Verification items for the finished model (mm, model axes). A direction names the side the tool comes from. Round coordinates to 2 decimals unless told otherwise and drop trailing zeros. Write each loop counter-clockwise with the first axis right and the second up, starting at its lowest first coordinate (ties: lowest second). Pieces come first, ordered by that corner, then holes. Notation, with made-up numbers: (-12.75, -24.5) - (16.25, -24.5) arc R29 cw to (16.25, -4.5) - close; hole circle Ø6 at (61, -39). An arc over 180 degrees is marked (long way). Answer as a JSON object with one key per item and string values.
```python
from build123d import *

# Parameters (mm, degrees)
F0_W     = 100.019608
F0_H     = 91
F2_DEPTH = 3
F3_DEPTH = 10
F4_R     = 8


with BuildPart() as f2:
    # F0 (on Front) → F2 (new body)
    with BuildSketch(Plane.XZ):
        with Locations((0, 25.5)):
            Rectangle(F0_W, F0_H)
        Polygon((0, 0), (-29.386316, 0), (-31.587102, -4.489604), (-32.485023, -4.049446), (-30.5, 0), (-31.613684, 0), (-35.009804, 0), (-35.009804, 1), (-30.009804, 1), (-5.990196, 50), (-10.5, 50), (-10.5, 51), (-5.5, 51), (-5.009804, 52), (-3.299214, 55.489604), (-2.401293, 55.049446), (-4.386316, 51), (0, 51), (4.386316, 51), (2.401293, 55.049446), (3.299214, 55.489604), (5.009804, 52), (5.5, 51), (10.5, 51), (10.5, 50), (5.990196, 50), (30.009804, 1), (35.009804, 1), (35.009804, 0), (31.613684, 0), (30.5, 0), (32.485023, -4.049446), (31.587102, -4.489604), (29.386316, 0), align=None, mode=Mode.SUBTRACT)
    extrude(amount=-F2_DEPTH)

    # F1 (on face) → F3 (join)
    with BuildSketch(Plane.XZ):
        with BuildLine():
            Line((-35.334654, -17), (-33.334654, -17))
            ThreePointArc((-33.334654, -17), (-35.804867, -5.945831), (-47.009804, -4.288724))
            Line((-47.009804, -4.288724), (-47.009804, -6.288724))
            ThreePointArc((-47.009804, -6.288724), (-37.230822, -7.34828), (-35.334654, -17))
        make_face()
        with BuildLine():
            ThreePointArc((-47.009804, 55.288724), (-35.804867, 56.945831), (-33.334654, 68))
            Line((-33.334654, 68), (-35.334654, 68))
            ThreePointArc((-35.334654, 68), (-37.230822, 58.34828), (-47.009804, 57.288724))
            Line((-47.009804, 57.288724), (-47.009804, 55.288724))
        make_face()
        with BuildLine():
            Line((35.334654, 68), (33.334654, 68))
            ThreePointArc((33.334654, 68), (35.804867, 56.945831), (47.009804, 55.288724))
            Line((47.009804, 55.288724), (47.009804, 57.288724))
            ThreePointArc((47.009804, 57.288724), (37.230822, 58.34828), (35.334654, 68))
        make_face()
        with BuildLine():
            ThreePointArc((47.009804, -4.288724), (35.804867, -5.945831), (33.334654, -17))
            Line((33.334654, -17), (35.334654, -17))
            ThreePointArc((35.334654, -17), (37.230822, -7.34828), (47.009804, -6.288724))
            Line((47.009804, -6.288724), (47.009804, -4.288724))
        make_face()
    extrude(amount=F3_DEPTH)

    # F4
    f4_edges = [f2.edges().sort_by_distance(p)[0] for p in [
        (-50.009804, 1.5, 71),
        (50.009804, 1.5, 71),
        (50.009804, 1.5, -20),
        (-50.009804, 1.5, -20),
    ]]
    fillet(f4_edges, radius=F4_R)


solid = f2.part
```
1. Cross-section at C-C (z = 47). Record the boundary of the cut face in (x, y).
Completed:
{"outline": "(-50.01, 0) - (-7.46, 0) - (-7.46, 3) - (-50.01, 3) - close; (7.46, 0) - (50.01, 0) - (50.01, 3) - (7.46, 3) - close"}
2. Access from +Z, -Z, +X, -X, +Y, -Y to the whole of each face (thin tool, end or side, straight path). Record for faces 1 (the face through (36.6, -10, -7.6)), 2 (the face through (35.93, -4.93, -5.83)), 3 (the face through (-31.506, 1.479, -2.053)).
Completed:
{"face 1": "+Z, -Z, +X, -X, -Y", "face 2": "-Y", "face 3": "+Y, -Y"}
3. Mould release check, pull along X, two halves, no side actions. Record for faces 4 (the face through (-47.73, 1.52, -17.59)), 5 (the face through (33, 1, 0)), 6 (the face through (-37, -10, -7)): released by +X, released by -X, zero draft, split by the parting line, or undercut.
Completed:
{"face 4": "released by -X", "face 5": "undercut", "face 6": "zero draft"}
4. Cross-section at A-A (y = -6.5). Record the boundary of the cut face in (x, z).
Completed:
{"outline": "(-47.01, -6.29) arc R8.3 cw to (-35.33, -17) - (-33.33, -17) arc R10 ccw to (-47.01, -4.29) - close; (-47.01, 55.29) arc R10 ccw to (-33.33, 68) - (-35.33, 68) arc R8.3 cw to (-47.01, 57.29) - close; (33.33, -17) - (35.33, -17) arc R8.3 cw to (47.01, -6.29) - (47.01, -4.29) arc R10 ccw to start; (33.33, 68) arc R10 ccw to (47.01, 55.29) - (47.01, 57.29) arc R8.3 cw to (35.33, 68) - close"}
5. Material ranges on probe 1 along Y at (x, z) = (29.5, 50); probe 2 along Z at (x, y) = (5, 0.75); probe 3 along X at (y, z) = (-1.75, -15), recorded low to high. Write a range as from..to.
Completed:
{"probe 1": "y = 0..3", "probe 2": "z = -20..0, 52.02..71", "probe 3": "x = -34.69..-32.76, 32.76..34.69"}
6. Go/stop test with flat-tipped pins: pin 1 (0.6 mm diameter, centred on y = -3.5, z = 56.5, fed in from -X); pin 2 (2 mm diameter, centred on y = -7.5, z = 56, fed in from +X); pin 3 (1.6 mm diameter, centred on x = -34, y = -6.5, fed in from -Z); pin 4 (3 mm diameter, centred on y = -0.5, z = -6.5, fed in from +X). Record where each tip stops, or that it passes through.
Completed:
{"pin 1": "stops at x = -47.01", "pin 2": "stops at x = 47.01", "pin 3": "stops at z = -17", "pin 4": "stops at x = 50.01"}
7. Cross-section at B-B (x = 25). Record the boundary of the cut face in (y, z), plus the area to 3 significant figures.
Completed:
{"outline": "(0, -20) - (3, -20) - (3, 0) - (0, 0) - close; (0, 11.22) - (3, 11.22) - (3, 71) - (0, 71) - close", "area": "239 mm^2"}
8. Cross-section at D-D (x = -40). Record the boundary of the cut face in (y, z), plus the area to 3 significant figures.
Completed:
{"outline": "(-10, -5.67) - (0, -5.67) - (0, -20) - (3, -20) - (3, 71) - (0, 71) - (0, 56.67) - (-10, 56.67) - (-10, 54.62) - (0, 54.62) - (0, -3.62) - (-10, -3.62) - close", "area": "314 mm^2"}
